Geometry: final body of the model. Coordinates: model frame, mm. A direction names the side the tool comes from. Give positions to 0.01 mm unless a question says otherwise; leave off trailing zeros. Write each loop counter-clockwise with the first axis right and the second up, starting at its lowest first coordinate (ties: lowest second). Pieces come first, ordered by that corner, then holes. Notation, with made-up numbers: (-10.75, -25.75) -> (17.25, -25.75) arc R21 ccw to (17.25, 4.25) -> close; hole circle Ø7 at (2.25, -12.75). An arc over 180 degrees is marked (long way). Use CSV: the item, a comma, the result in double quotes. Start each with the question number.
1) Section C-C (z = 4.75). Output: boundary loops of the cut face in (x, y), plus the area to 3 significant figures.
2) Set-up query: faces 1 (the face through (-1.5, 0.07, 10.99)), 2 (the face through (0, -1, 5)). Return all of +Z, -Z, +X, -X, +Y, -Y with unobstructed straight access to the full face (end or side cutting, diameter ignored); none if empty.
3) Material intervals for line 1 (Z direction, x = 0.75, y = -0.7); line 2 (Y direction, x = 0, z = 5.25); line 3 (X direction, y = 0.9, z = 10.75), sorted ascending. Write a range as [from, to].
4) Section A-A (x = 0). Output: boundary loops of the cut face in (y, z), plus the area to 3 significant figures.
5) Contact query for a flat-ended pin moving along its axis: P1, Ø1.5, axis at y = 0.5, z = 5, coming from the +X side. Output: stop coordinate, or through.
6) Section D-D (y = -1.15). Output: boundary loops of the cut face in (x, z), plus the area to 3 significant figures.
```python
from build123d import *

# Parameters (mm, degrees)
CROQUIS1_R              = 1
SALIENTE_EXTRUIR1_DEPTH = 10
CHAFL_N1_SIZE           = 0.2
CROQUIS2_R              = 1.5
SALIENTE_EXTRUIR2_DEPTH = 2


with BuildPart() as part:
    # Croquis1 → Saliente-Extruir1 (new body)
    with BuildSketch(Plane.XY):
        Circle(CROQUIS1_R)
    extrude(amount=SALIENTE_EXTRUIR1_DEPTH)

    # Chaflán1
    chafl_n1_edges = [part.edges().sort_by_distance(p)[0] for p in [
        (-1, 0, 0),
    ]]
    chamfer(chafl_n1_edges, length=CHAFL_N1_SIZE)

    # Croquis2 → Saliente-Extruir2 (add)
    with BuildSketch(Plane.XY.offset(10)):
        Circle(CROQUIS2_R)
    extrude(amount=SALIENTE_EXTRUIR2_DEPTH)


solid = part.part
```
Answers follow:
1,outline,"circle Ø2 at (0, 0)"
1,area,"3.14 mm^2"
2,face 1,"+Z, -Z"
2,face 2,"-Z"
3,line 1,"z = [10, 12]"
3,line 2,"y = [-1, 1]"
3,line 3,"x = [-1.2, 1.2]"
4,outline,"(-1.5, 10) -> (-1, 10) -> (-1, 0.2) -> (-0.8, 0) -> (0.8, 0) -> (1, 0.2) -> (1, 10) -> (1.5, 10) -> (1.5, 12) -> (-1.5, 12) -> close"
4,area,"26.0 mm^2"
5,P1,"stops at x = 1"
6,outline,"(-0.96, 10) -> (0.96, 10) -> (0.96, 12) -> (-0.96, 12) -> close"
6,area,"3.85 mm^2"
